Autodesk Inventor part; units mm, degrees
ref_plane "YZ Plane" through (0, 0, 0) normal (1, 0, 0) x (0, 1, 0)
ref_plane "XZ Plane" through (0, 0, 0) normal (0, 1, 0) x (-1, 0, 0)
ref_plane "XY Plane" through (0, 0, 0) normal (0, 0, 1) x (1, 0, 0)
sketch "スケッチ1" plane through (0, 0, 0) normal (0, 1, 0) x (-1, 0, 0)
  line L0 (-40, -39) -> (40, -39)
  line L1 (40, -39) -> (40, 39)
  line L2 (40, 39) -> (-40, 39)
  line L3 (-40, 39) -> (-40, -39)
  line L4 (-40, -39) -> (40, 39) construction
  line L5 (40, -39) -> (-40, 39) construction
  point P0 (0, 0)
  dimension "d0" = 80
  dimension "d1" = 78
extrude "押し出し1" add sketch "スケッチ1" along normal blind 3
sketch "スケッチ2" plane through (0, 3, 0) normal (0, 1, 0) x (1, 0, 0)
  line L0 (34, 30) -> (-34, 30)
  line L1 (-34, 30) -> (-34, -30)
  line L2 (-34, -30) -> (34, -30)
  line L3 (34, -30) -> (34, 30)
  line L4 (34, 30) -> (-34, -30) construction
  line L5 (-34, 30) -> (34, -30) construction
  point P0 (0, 0)
  dimension "d4" = 68
  dimension "d5" = 60
hole "穴1" at (-34, 3, 30) at (34, 3, 30) at (34, 3, -30) at (-34, 3, -30) direction (0, -1, 0) diameter 5.2 depth 8 tip angle 118
sketch "スケッチ3" plane through (0, 3, 0) normal (0, 1, 0) x (1, 0, 0)
  line L0 (13.5, 25) -> (-13.5, 25)
  line L1 (-13.5, 25) -> (-13.5, -25)
  line L2 (-13.5, -25) -> (13.5, -25)
  line L3 (13.5, -25) -> (13.5, 25)
  line L4 (13.5, 25) -> (-13.5, -25) construction
  line L5 (-13.5, 25) -> (13.5, -25) construction
  point P0 (0, 0)
  dimension "d13" = 27
  dimension "d14" = 50
hole "穴2" at (-13.5, 3, 25) at (13.5, 3, 25) at (13.5, 3, -25) at (-13.5, 3, -25) direction (0, -1, 0) diameter 5.3 depth 8 tip angle 118 countersink diameter 11 countersink angle 90
chamfer "面取り1" distance 5 angle 45 4 edges at (-40, 1.5, 39) (40, 1.5, 39) (40, 1.5, -39) (-40, 1.5, -39)
fillet "フィレット3" radius 2 8 edges at (-35, 1.5, 39) (35, 1.5, 39) (40, 1.5, 34) (40, 1.5, -34) (35, 1.5, -39) (-40, 1.5, -34) (-35, 1.5, -39) (-40, 1.5, 34)
properties part number "CCM_Mount_A"
Geometry: final body of the model. Coordinates: model frame, mm. Round coordinates to 2 decimals unless told otherwise and drop trailing zeros. Loops run counter-clockwise (first coordinate to the right, second up) from the corner with the lowest first, then second, coordinate; pieces in that order, holes last. Notation, with made-up numbers: (85, -31.75) -> (92, -31.75) arc R20 ccw to (92, 6.25) -> close; hole circle Ø5 at (-30.5, 69.5). An arc over 180 degrees is marked (long way). One line per question, with ' | ' between items. Start each with the question number.
1. Section B-B on x = -13.5. Output: boundary loops of the cut face in (y, z).
2. Line query: line 1 along X through (y, z) = (2.4, 30); line 2 along X through (y, z) = (0.05, -25); line 3 along Z through (x, y) = (-34, 1.15). Output: solid intervals per line, ascending. Write a range as [from, to].
3. Mould query, pull axis X, two halves, no side actions, for faces 1 (the face through (33.9, 1.5, -32.6)), 2 (the face through (-38, 1, 36)), 3 (the face through (12.417, 0.328, 27.613)), 4 (the face through (37, 2, -37)). Classes: pulls with the +X half, pulls with the -X half, needs draft (parallel to the pull), parting line crosses it, or undercut.
4. Section A-A on y = 1.55. Count the separate pieces of the cut face and the enclosed holes in it, and give its area (3 significant figures).
Returned:
1) outline: (0, -39) -> (3, -39) -> (3, -30.5) -> (0.15, -27.65) -> (0, -27.65) -> close; (0, -22.35) -> (0.15, -22.35) -> (3, -19.5) -> (3, 19.5) -> (0.15, 22.35) -> (0, 22.35) -> close; (0, 27.65) -> (0.15, 27.65) -> (3, 30.5) -> (3, 39) -> (0, 39) -> close
2) line 1: x = [-40, -36.6], [-31.4, 31.4], [36.6, 40] | line 2: x = [-40, -16.15], [-10.85, 10.85], [16.15, 40] | line 3: z = [-39, -32.6], [-27.4, 27.4], [32.6, 39]
3) face 1: undercut | face 2: pulls with the -X half | face 3: undercut | face 4: pulls with the +X half
4) separate pieces: 1 | enclosed holes: 8 | area: 5,900 mm2
